from build123d import *

# Parameters (mm, degrees)
F0_W     = 7.95
F0_H     = 4
F1_DEPTH = 10
F2_R     = 2.6
F3_DEPTH = 21
F4_R     = 2.6
F5_DEPTH = 50
F6_R     = 3


with BuildPart() as f1:
    # F0 (on Top) → F1 (new body)
    with BuildSketch(Plane.XY):
        with BuildLine():
            Line((24.738697, 12.982003), (13.873269, 12.982003))
            ThreePointArc((13.873269, 12.982003), (12.462028, 14.342171), (10.918168, 15.549714))
            Line((10.918168, 15.549714), (10.918168, 32))
            Line((10.918168, 32), (4.018168, 32))
            Line((4.018168, 32), (4.018168, 20))
            Line((4.018168, 20), (-3.181832, 20))
            Line((-3.181832, 20), (-3.181832, 32))
            Line((-3.181832, 32), (-10.081832, 32))
            Line((-10.081832, 32), (-10.081832, 16.104554))
            ThreePointArc((-10.081832, 16.104554), (-19, 0), (-10.081832, -16.104554))
            ThreePointArc((-10.081832, -16.104554), (-6.760669, -17.756502), (-3.181832, -18.731683))
            ThreePointArc((-3.181832, -18.731683), (0.425887, -18.995226), (4.018168, -18.570254))
            ThreePointArc((4.018168, -18.570254), (7.26281, -17.557095), (10.274998, -15.982003))
            Line((10.274998, -15.982003), (10.918168, -15.982003))
            Line((10.918168, -15.982003), (12.699907, -15.982003))
            Line((12.699907, -15.982003), (24.738697, -15.982003))
            Line((24.738697, -15.982003), (24.738697, -7.982003))
            Line((24.738697, -7.982003), (12.699907, -7.982003))
            ThreePointArc((12.699907, -7.982003), (-15, 0), (12.699907, 7.982003))
            Line((12.699907, 7.982003), (24.738697, 7.982003))
            Line((24.738697, 7.982003), (24.738697, 12.982003))
        make_face()
        with Locations((18.763697, -11.982003)):
            Rectangle(F0_W, F0_H, mode=Mode.SUBTRACT)
        with BuildLine():
            Line((10.918168, -32), (10.918168, -15.982003))
            Line((10.918168, -15.982003), (10.274998, -15.982003))
            ThreePointArc((10.274998, -15.982003), (7.26281, -17.557095), (4.018168, -18.570254))
            Line((4.018168, -18.570254), (4.018168, -20))
            Line((4.018168, -20), (4.018168, -32))
            Line((4.018168, -32), (10.918168, -32))
        make_face()
        with BuildLine():
            ThreePointArc((-3.181832, -18.731683), (-6.760669, -17.756502), (-10.081832, -16.104554))
            Line((-10.081832, -16.104554), (-10.081832, -32))
            Line((-10.081832, -32), (-3.181832, -32))
            Line((-3.181832, -32), (-3.181832, -20))
            Line((-3.181832, -20), (-3.181832, -18.731683))
        make_face()
        with BuildLine():
            ThreePointArc((4.018168, -18.570254), (0.425887, -18.995226), (-3.181832, -18.731683))
            Line((-3.181832, -18.731683), (-3.181832, -20))
            Line((-3.181832, -20), (4.018168, -20))
            Line((4.018168, -20), (4.018168, -18.570254))
        make_face()
    extrude(amount=F1_DEPTH)

    # F2 (on face) → F3 (cut, through all)
    with BuildSketch(Plane.YZ.offset(10.918168)):
        with BuildLine():
            ThreePointArc((32, 5), (30.535534, 1.464466), (27, 0))
            Line((27, 0), (32, 0))
            Line((32, 0), (32, 5))
        make_face()
        with BuildLine():
            ThreePointArc((27, 10), (30.535534, 8.535534), (32, 5))
            Line((32, 5), (32, 10))
            Line((32, 10), (27, 10))
        make_face()
        with Locations((27, 5)):
            Circle(F2_R)
    extrude(amount=-F3_DEPTH, mode=Mode.SUBTRACT)

    # F4 (on face) → F5 (cut, symmetric)
    with BuildSketch(Plane(origin=(0, -13.982003, 0), x_dir=(-1, 0, 0), z_dir=(0, 1, 0))):
        with Locations((-18.763697, 5)):
            Circle(F4_R)
    extrude(amount=F5_DEPTH, both=True, mode=Mode.SUBTRACT)

    # F6
    f6_edges = [f1.edges().sort_by_distance(p)[0] for p in [
        (24.738697, 12.982003, 5),
        (24.738697, -7.982003, 5),
        (24.738697, -15.982003, 5),
    ]]
    fillet(f6_edges, radius=F6_R)


solid = f1.part
Could you check a few things on this model? Use its own coordinates, in mm. A direction names the side the tool comes from. Coordinates: 2 decimals unless noted, no trailing zeros. Write each loop counter-clockwise with the first axis right and the second up, starting at its lowest first coordinate (ties: lowest second). Pieces come first, ordered by that corner, then holes. Notation, with made-up numbers: M -32.5,40.5 L 16.5,40.5 A15 ccw 16.5,59.5 Z; hole C 47.5,-25 d6. An arc over 180 degrees is marked long. One line per question, with ' | ' between items.
1) For faces 1 (the face through (10.918, 22, 5)), 2 (the face through (23.8, -8.8, 5.1)), 3 (the face through (15, -15.982, 5)), 4 (the face through (16, -13.982, 5)), which set-ups out of +Z, -Z, +X, -X, +Y, -Y let a thin tool reach every point of the face, with its end or its side?
Checks:
face 1: +Z, -Z, +X, +Y | face 2: +Z, -Z, +X | face 3: +Z, -Z, +X, -Y | face 4: +Z, -Z
2) Imagine slicing it at A-A, the plane x = 9.5. Write out the boundary of the cut face in (y, z), and give its area (3 significant figures).
Checks:
outline: M -32,0 L -11.61,0 L -11.61,10 L -32,10 Z; M 11.61,0 L 27,0 A5 ccw 27,10 L 11.61,10 Z; hole C 27,5 d5.2 | area: 376 mm²
3) Imagine slicing it at B-B, the plane y = -26. Write out the boundary of the cut face in (x, z), and give its area (3 significant figures).
Checks:
outline: M -10.08,0 L -3.18,0 L -3.18,10 L -10.08,10 Z; M 4.02,0 L 10.92,0 L 10.92,10 L 4.02,10 Z | area: 138 mm²
4) For pin 1 Ø3 at (y, z) = (-21.5, 7) entering from -X; pin 2 Ø4 at (x, z) = (18, 6) entering from +Y; pin 3 Ø10 at (x, y) = (15.5, -1) entering from +Z; pin 4 Ø5 at (y, z) = (24, 7) entering from +X, each with a flat end and sliding along its axis, tell me the tip position at first contact or that it passes through.
Checks:
pin 1: x = -10.08 | pin 2: y = 12.98 | pin 3: through | pin 4: x = 10.92
5) Imagine slicing it at C-C, the plane x = 0. Write out the boundary of the cut face in (y, z), and give its area (4 significant figures).
Checks:
outline: M -20,0 L -15,0 L -15,10 L -20,10 Z; M 15,0 L 20,0 L 20,10 L 15,10 Z | area: 100.0 mm²
6) I need wall thicknesses on probe 1 along Y at (x, z) = (21.5, 3.5); probe 2 along X at (y, z) = (-28, 2); probe 3 along Y at (x, z) = (0, 7.25). Which ranges of each line are inside material? Lowest first, please. Write a range as [from, to].
Checks:
probe 1: [-15.98, -13.98], [-9.98, -7.98], [7.98, 12.98] | probe 2: [-10.08, -3.18], [4.02, 10.92] | probe 3: [-20, -15], [15, 20]
7) If we mould it in two halves opening along Y, with no side actions, what happens to faces 5 (the face through (-14.99, -0.54, 4.93)), 6 (the face through (22.739, -12, 5)), 7 (the face through (7, -32, 5)), 8 (the face through (4.018, 23, 5))? For each: released by +Y, released by -Y, zero draft, split by the parting line, or undercut.
Checks:
face 5: undercut | face 6: undercut | face 7: released by -Y | face 8: zero draft
